```python
from build123d import *

# Parameters (mm, degrees)
SKETCH1_R           = 1.3462
SKETCH1_W           = 5.4034
SKETCH1_H           = 22.6066
SKETCH1_W_2         = 60.6932
SKETCH1_H_2         = 7.81
SKETCH1_W_3         = 5.588
SKETCH1_H_3         = 23.368
BOSS_EXTRUDE1_DEPTH = 3.048


with BuildPart() as part:
    # Sketch1 → Boss-Extrude1 (new body)
    with BuildSketch(Plane.XY):
        with BuildLine():
            Line((57.404932375, 30.507694304), (-34.084892625, 30.507694304))
            ThreePointArc((-34.084892625, 30.507694304), (-36.778969461, 29.391771141), (-37.894892625, 26.697694304))
            Line((-37.894892625, 26.697694304), (-37.894892625, -32.641005696))
            ThreePointArc((-37.894892625, -32.641005696), (-36.778969461, -35.335082532), (-34.084892625, -36.451005696))
            Line((-34.084892625, -36.451005696), (-23.844892625, -33.084405696))
            Line((-23.844892625, -33.084405696), (28.474307375, -33.084405696))
            Line((28.474307375, -33.084405696), (38.714307375, -36.451005696))
            Line((38.714307375, -36.451005696), (57.405007375, -36.451005696))
            ThreePointArc((57.405007375, -36.451005696), (60.108826144, -35.325305244), (61.214907375, -32.613401529))
            Line((61.214907375, -32.613401529), (61.214907375, -28.627805696))
            Line((61.214907375, -28.627805696), (35.575007375, -28.627805696))
            Line((35.575007375, -28.627805696), (35.575007375, -12.628005696))
            Line((35.575007375, -12.628005696), (56.975007375, -12.628005696))
            Line((56.975007375, -12.628005696), (56.975007375, -9.121805696))
            Line((56.975007375, -9.121805696), (40.325007375, -9.121805696))
            Line((40.325007375, -9.121805696), (40.325007375, 4.997894304))
            Line((40.325007375, 4.997894304), (56.975007375, 4.997894304))
            Line((56.975007375, 4.997894304), (56.975007375, 8.658194304))
            Line((56.975007375, 8.658194304), (40.325007375, 8.658194304))
            Line((40.325007375, 8.658194304), (40.325007375, 24.068294304))
            Line((40.325007375, 24.068294304), (61.214907375, 24.068294304))
            Line((61.214907375, 24.068294304), (61.214907375, 26.683892153))
            ThreePointArc((61.214907375, 26.683892153), (60.103884597, 29.386886916), (57.404932375, 30.507694304))
        make_face()
        with Locations(Location((57.405007375, -32.641005696, 0), (0, 0, 180))):
            Circle(SKETCH1_R, mode=Mode.SUBTRACT)
        with Locations(Location((-34.084892625, -32.641005696, 0), (0, 0, 180))):
            Circle(SKETCH1_R, mode=Mode.SUBTRACT)
        with Locations(Location((-34.084892625, 26.697694304, 0), (0, 0, 180))):
            Circle(SKETCH1_R, mode=Mode.SUBTRACT)
        with Locations(Location((57.404932375, 26.697694304, 0), (0, 0, 180))):
            Circle(SKETCH1_R, mode=Mode.SUBTRACT)
        with Locations((16.546707375, -19.663505696)):
            Rectangle(SKETCH1_W, SKETCH1_H, mode=Mode.SUBTRACT)
        with Locations((1.341707375, 21.991994304)):
            Rectangle(SKETCH1_W_2, SKETCH1_H_2, mode=Mode.SUBTRACT)
        with Locations((-26.210892625, -1.882805696)):
            Rectangle(SKETCH1_W_3, SKETCH1_H_3, mode=Mode.SUBTRACT)
    extrude(amount=BOSS_EXTRUDE1_DEPTH)


solid = part.part
```
CAD build for the part. Positions are in the model's coordinates, mm. A direction names the side the tool comes from. Round coordinates to 2 decimals unless told otherwise and drop trailing zeros. Loops run counter-clockwise (first coordinate to the right, second up) from the corner with the lowest first, then second, coordinate; pieces in that order, holes last. Notation, with made-up numbers: M -10.75,58 L 35.25,58 A36 ccw 35.25,92 Z; hole C -18,79.25 d5. An arc over 180 degrees is marked long. Use a Markdown table: item, result. Add a question column.
(1) Which spindle directions (+Z, -Z, +X, -X, +Y, -Y) get a long thin tool onto all of the face, cutting with end or side? Do faces 4 (the face through (51, 24.068, 2)), 5 (the face through (48, -36.451, 2)), 6 (the face through (-29.005, 22, 2)). Say none if no direction does.
(2) Cut at D-D (y = 22.5). Give the cut face in (x, z) (3 decimals).
(3) Flat gauge pins, fed straight in: pin 1 (0.9 mm diameter, centred on x = 15, z = 2, fed in from -Y); pin 2 (1.5 mm diameter, centred on y = 16.5, z = 1, fed in from +X) (3 decimals); pin 3 (0.9 mm diameter, centred on y = -10, z = 1, fed in from +X) (3 decimals). Where does each tip first touch, or does it go through?
(4) Pull direction X, two halves, no side cores. Call faces 1 (the face through (13.845, -20, 2)), 2 (the face through (60.13, 29.36, 1.5)), 3 (the face through (12, 30.508, 2)): +X half, -X half, draft (parallel to the pull), parting line (faces both ways), or undercut.
(5) Cut at C-C (x = 45.5). Give the cut face in (y, z), and give its area (3 significant figures).
(6) Cut at A-A (y = 1). Give the cut face in (x, z) (3 decimals).
(7) Cut at B-B (x = 15). Give the cut face in (y, z), and give its area (3 significant figures).
(8) Drill centre lines: line 1 (Y direction, x = 55, z = 2.75); line 2 (Y direction, x = 18.5, z = 2.8); line 3 (Y direction, x = -23.5, z = 2.45). Where is each one in solid material? Low to high.
Geometry says:
| question | item | result |
|---|---|---|
| 1 | face 4 | +Z, -Z, +X |
| 1 | face 5 | +Z, -Z, +X, -X, -Y |
| 1 | face 6 | +Z, -Z |
| 2 | outline | M -37.895,0 L -29.005,0 L -29.005,3.048 L -37.895,3.048 Z; M 31.688,0 L 40.325,0 L 40.325,3.048 L 31.688,3.048 Z |
| 3 | pin 1 | stops at y = -33.08 |
| 3 | pin 2 | stops at x = 40.325 |
| 3 | pin 3 | stops at x = 56.975 |
| 4 | face 1 | undercut |
| 4 | face 2 | +X half |
| 4 | face 3 | draft |
| 5 | outline | M -36.45,0 L -28.63,0 L -28.63,3.05 L -36.45,3.05 Z; M -12.63,0 L -9.12,0 L -9.12,3.05 L -12.63,3.05 Z; M 5,0 L 8.66,0 L 8.66,3.05 L 5,3.05 Z; M 24.07,0 L 30.51,0 L 30.51,3.05 L 24.07,3.05 Z |
| 5 | area | 65.3 mm² |
| 6 | outline | M -37.895,0 L -29.005,0 L -29.005,3.048 L -37.895,3.048 Z; M -23.417,0 L 40.325,0 L 40.325,3.048 L -23.417,3.048 Z |
| 7 | outline | M -33.08,0 L -30.97,0 L -30.97,3.05 L -33.08,3.05 Z; M -8.36,0 L 18.09,0 L 18.09,3.05 L -8.36,3.05 Z; M 25.9,0 L 30.51,0 L 30.51,3.05 L 25.9,3.05 Z |
| 7 | area | 101 mm² |
| 8 | line 1 | y = -36.45 to -28.63, -12.63 to -9.12, 5 to 8.66, 24.07 to 30.51 |
| 8 | line 2 | y = -33.08 to -30.97, -8.36 to 18.09, 25.9 to 30.51 |
| 8 | line 3 | y = -33.08 to -13.57, 9.8 to 18.09, 25.9 to 30.51 |
